from build123d import *

# Parameters (mm, degrees)
F0_R     = 16.5
F1_DEPTH = 8
F2_R     = 1.05
F3_DEPTH = 2.5
F4_R     = 1
F5_DEPTH = 2.5


with BuildPart() as f1:
    # F0 (on Top) → F1 (new body)
    with BuildSketch(Plane.XY):
        Circle(F0_R)
    extrude(amount=F1_DEPTH)

    # F2 (on face) → F3 (cut)
    with BuildSketch(Plane(origin=(0, 0, 0), x_dir=(1, 0, 0), z_dir=(0, 0, -1))):
        with Locations((0, 15.05)):
            Circle(F2_R)
        with Locations((15, 0.05)):
            Circle(F2_R)
        with Locations((0, -14.95)):
            Circle(F2_R)
    extrude(amount=-F3_DEPTH, mode=Mode.SUBTRACT)

    # F4 (on face) → F5 (join)
    with BuildSketch(Plane.XY.offset(8)):
        with Locations((0, 15)):
            Circle(F4_R)
        with Locations((15, 0)):
            Circle(F4_R)
        with Locations((0, -15)):
            Circle(F4_R)
    extrude(amount=F5_DEPTH)


solid = f1.part
Source: CAD feature listing. Evaluate the final solid. Frame: model axes, mm. A direction names the side the tool comes from. Round coordinates to 2 decimals unless told otherwise and drop trailing zeros. Write each loop counter-clockwise with the first axis right and the second up, starting at its lowest first coordinate (ties: lowest second). Pieces come first, ordered by that corner, then holes. Notation, with made-up numbers: (-26, 37.25) - (-15, 37.25) arc R20 cw to (-15, 74.25) - close; hole circle Ø11 at (-15, 7). An arc over 180 degrees is marked (long way). Use CSV: the item, a comma, the result in double quotes. Start each with the question number.
(1) Mould query, pull axis Y, two halves, no side actions, for faces 1 (the face through (15, 0, 10.5)), 2 (the face through (16, 0, 9)), 3 (the face through (0, -16, 9)). Classes: pulls with the +Y half, pulls with the -Y half, needs draft (parallel to the pull), parting line crosses it, or undercut.
(2) Cut plane C-C, the plane z = 1.25. Return loops of the section in (x, y).
(3) Cut plane D-D, the plane y = -8. Return loops of the section in (x, z).
(4) Cut plane A-A, the plane x = 0. Return loops of the section in (y, z).
(5) Material intervals for probe 1 along Y at (x, z) = (0, 1.4); probe 2 along Y at (x, z) = (-0.5, 1); probe 3 along Z at (x, y) = (-6.5, 8), sorted ascending. Write a range as [from, to].
(6) Set-up query: faces 4 (the face through (0, -14, 1)), 5 (the face through (0, -15, 10.5)), 6 (the face through (0, 14, 9)). Return all of +Z, -Z, +X, -X, +Y, -Y with unobstructed straight access to the full face (end or side cutting, diameter ignored); none if empty.
(7) First-contact query: pin 1 Ø4 at (y, z) = (-10, 8.5) entering from -X; pin 2 Ø1 at (x, y) = (-3, 12) entering from +Z; pin 3 Ø1 at (x, y) = (15, -0.5) entering from -Z. Flat tips, straight axial feed; report the tip coordinate or a pass-through.
(8) Cut plane B-B, the plane z = 8.5. Return loops of the section in (x, y).
Geometry says:
1,face 1,"needs draft"
1,face 2,"parting line crosses it"
1,face 3,"undercut"
2,outline,"circle Ø33 at (0, 0); hole circle Ø2.1 at (0, -15.05); hole circle Ø2.1 at (0, 14.95); hole circle Ø2.1 at (15, -0.05)"
3,outline,"(-14.43, 0) - (14.43, 0) - (14.43, 8) - (-14.43, 8) - close"
4,outline,"(-16.5, 0) - (-16.1, 0) - (-16.1, 2.5) - (-14, 2.5) - (-14, 0) - (13.9, 0) - (13.9, 2.5) - (16, 2.5) - (16, 0) - (16.5, 0) - (16.5, 8) - (16, 8) - (16, 10.5) - (14, 10.5) - (14, 8) - (-14, 8) - (-14, 10.5) - (-16, 10.5) - (-16, 8) - (-16.5, 8) - close"
5,probe 1,"[-16.5, -16.1], [-14, 13.9], [16, 16.5]"
5,probe 2,"[-16.49, -15.97], [-14.13, 14.03], [15.87, 16.49]"
5,probe 3,"[0, 8]"
6,face 4,"-Z"
6,face 5,"+Z, +X, -X, +Y, -Y"
6,face 6,"+Z"
7,pin 1,"x = -14.4"
7,pin 2,"z = 8"
7,pin 3,"z = 2.5"
8,outline,"circle Ø2 at (0, -15); circle Ø2 at (0, 15); circle Ø2 at (15, 0)"
